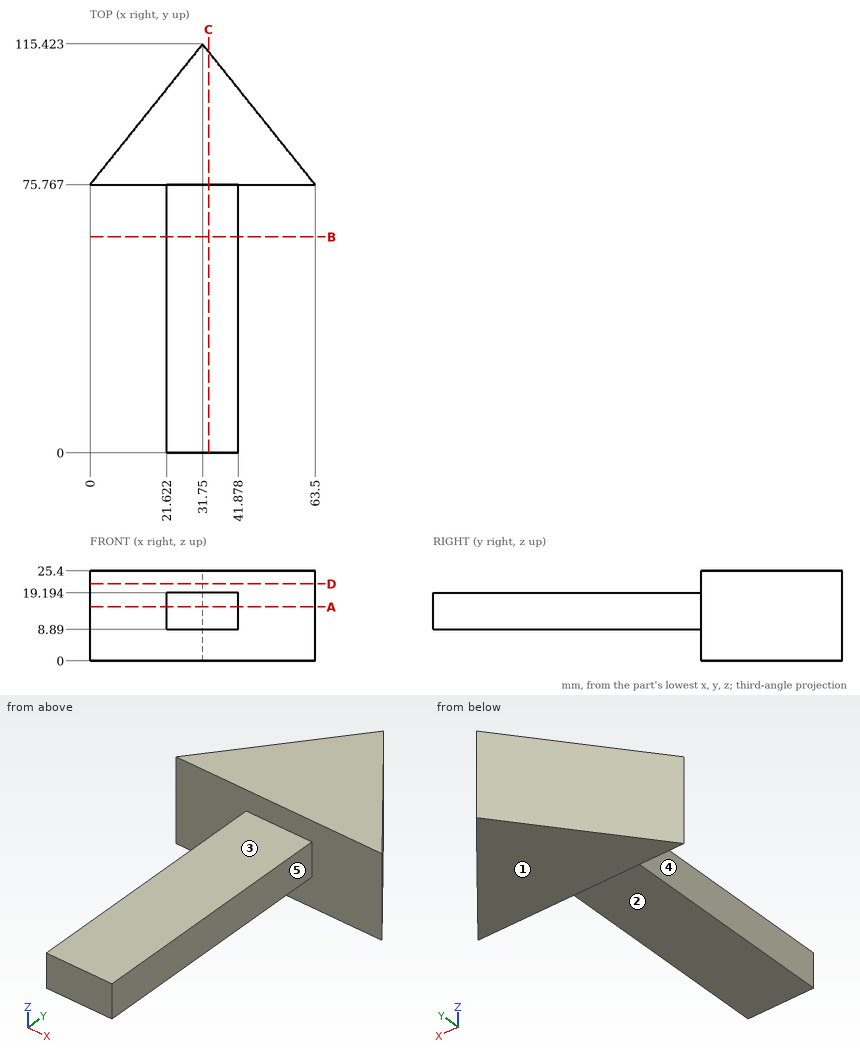
Geometry: see drawing. Coordinates: mm, zero at the bounding-box minimum. A direction names the side the tool comes from. Coordinates: 2 decimals unless noted, no trailing zeros. Order: outer loops, then holes, each group sorted by start corner. A loop starts at its lowest first (then second) coordinate and runs counter-clockwise, first axis right, second up. Notation, with made-up numbers: (-9.75, 84.5) - (48.25, 84.5) arc R26 cw to (48.25, 120.5) - close; hole circle Ø9 at (19, -24.75). An arc over 180 degrees is marked (long way). Write each question's results on one line, items separated by ' | '.
1) Line query: line 1 (Z direction, x = 23, y = 48.5) (1 decimal); line 2 (X direction, y = 9, z = 12.5); line 3 (Y direction, x = 30, z = 12) (1 decimal). Output: solid intervals per line, ascending. Write a range as from..to.
Results list:
line 1: 8.9..19.2 | line 2: 21.62..41.88 | line 3: 0..113.2
2) Pin query (flat end, axial travel): pin 1 (11.5 mm diameter, centred on y = 52, z = 16, fed in from -X); pin 2 (10 mm diameter, centred on x = 17, y = 55, fed in from -Z); pin 3 (12 mm diameter, centred on x = 55, z = 9, fed in from -Y); pin 4 (6 mm diameter, centred on y = 61.5, z = 3.5, fed in from +X). Return the tip coordinate at first contact, or that it passes through.
Results list:
pin 1: x = 21.62 | pin 2: z = 8.89 | pin 3: y = 75.77 | pin 4: through
3) Set-up query: the marked faces 1, 2, 3, 4 and 5. Return all of +Z, -Z, +X, -X, +Y, -Y with unobstructed straight access to the full face (end or side cutting, diameter ignored); none if empty.
Results list:
face 1: -Z, +X, -X, +Y, -Y | face 2: -Z, +X, -X, -Y | face 3: +Z, +X, -X, -Y | face 4: +Z, -Z, -X, -Y | face 5: +Z, -Z, +X, -Y
4) Section A-A, the plane z = 15.25. Return loops of the section in (x, y).
Results list:
outline: (0, 75.77) - (21.62, 75.77) - (21.62, 0) - (41.88, 0) - (41.88, 75.77) - (63.5, 75.77) - (31.75, 115.42) - close
5) Section B-B, the plane y = 61. Return loops of the section in (x, z) (1 decimal), plus the area to 3 significant figures.
Results list:
outline: (21.6, 8.9) - (41.9, 8.9) - (41.9, 19.2) - (21.6, 19.2) - close | area: 209 mm^2
6) Section D-D, the plane z = 21.75. Return loops of the section in (x, y).
Results list:
outline: (0, 75.77) - (63.5, 75.77) - (31.75, 115.42) - close
7) Section C-C, the plane x = 33.5. Return loops of the section in (y, z) (1 decimal), plus the area to 3 significant figures.
Results list:
outline: (0, 8.9) - (75.8, 8.9) - (75.8, 0) - (113.2, 0) - (113.2, 25.4) - (75.8, 25.4) - (75.8, 19.2) - (0, 19.2) - close | area: 1,730 mm^2
